```python
from build123d import *

# Parameters (mm, degrees)
F1_DEPTH  = 70
F3_DEPTH  = 10
F4_R      = 6.5
F4_R_2    = 3.35
F5_DEPTH  = 4.1439934524
F6_R      = 6.5
F6_R_2    = 3.35
F7_DEPTH  = 4.1439934524
F8_R      = 6.5
F8_R_2    = 3.35
F9_DEPTH  = 4.1439934524
F10_R     = 6.5
F10_R_2   = 3.35
F11_DEPTH = 4.1439934524
F12_R     = 5
F12_R_2   = 4.1
F13_DEPTH = 10


with BuildPart() as f1:
    # F0 (on Top) → F1 (new body)
    with BuildSketch(Plane.XY):
        with BuildLine():
            Line((17.5, 66.7439135802), (-17.5, 66.7439135802))
            ThreePointArc((-17.5, 66.7439135802), (-48.7903679019, 48.7903679019), (-66.7439135802, 17.5))
            Line((-66.7439135802, 17.5), (-66.7439135802, -17.5))
            ThreePointArc((-66.7439135802, -17.5), (-48.7903679019, -48.7903679019), (-17.5, -66.7439135802))
            Line((-17.5, -66.7439135802), (17.5, -66.7439135802))
            ThreePointArc((17.5, -66.7439135802), (48.7903679019, -48.7903679019), (66.7439135802, -17.5))
            Line((66.7439135802, -17.5), (66.7439135802, 17.5))
            ThreePointArc((66.7439135802, 17.5), (48.7903679019, 48.7903679019), (17.5, 66.7439135802))
        make_face()
        with BuildLine():
            ThreePointArc((-62.5999201277, 17.5), (-45.9619407771, 45.9619407771), (-17.5, 62.5999201277))
            Line((-17.5, 62.5999201277), (17.5, 62.5999201277))
            ThreePointArc((17.5, 62.5999201277), (45.9619407771, 45.9619407771), (62.5999201277, 17.5))
            Line((62.5999201277, 17.5), (62.5999201277, -17.5))
            ThreePointArc((62.5999201277, -17.5), (45.9619407771, -45.9619407771), (17.5, -62.5999201277))
            Line((17.5, -62.5999201277), (-17.5, -62.5999201277))
            ThreePointArc((-17.5, -62.5999201277), (-45.9619407771, -45.9619407771), (-62.5999201277, -17.5))
            Line((-62.5999201277, -17.5), (-62.5999201277, 17.5))
        make_face(mode=Mode.SUBTRACT)
    extrude(amount=F1_DEPTH)

    # F2 (on face) → F3 (join)
    with BuildSketch(Plane.XY.offset(70)):
        with BuildLine():
            Line((17.5, 71.3862731903), (-17.5, 71.3862731903))
            ThreePointArc((-17.5, 71.3862731903), (-51.9723484172, 51.9723484172), (-71.3862731903, 17.5))
            Line((-71.3862731903, 17.5), (-71.3862731903, -17.5))
            ThreePointArc((-71.3862731903, -17.5), (-51.9723484172, -51.9723484172), (-17.5, -71.3862731903))
            Line((-17.5, -71.3862731903), (17.5, -71.3862731903))
            ThreePointArc((17.5, -71.3862731903), (51.9723484172, -51.9723484172), (71.3862731903, -17.5))
            Line((71.3862731903, -17.5), (71.3862731903, 17.5))
            ThreePointArc((71.3862731903, 17.5), (51.9723484172, 51.9723484172), (17.5, 71.3862731903))
        make_face()
    extrude(amount=F3_DEPTH)

    # F4 (on face) → F5 (cut, through all)
    with BuildSketch(Plane.XZ.offset(66.7439135802)):
        with Locations((0, 53)):
            Circle(F4_R)
        with Locations((0, 34)):
            Circle(F4_R_2)
        with Locations((0, 17)):
            Circle(F4_R_2)
    extrude(amount=-F5_DEPTH, mode=Mode.SUBTRACT)

    # F6 (on face) → F7 (cut, through all)
    with BuildSketch(Plane.YZ.offset(66.7439135802)):
        with Locations((0, 53)):
            Circle(F6_R)
        with Locations((0, 34)):
            Circle(F6_R_2)
        with Locations((0, 17)):
            Circle(F6_R_2)
    extrude(amount=-F7_DEPTH, mode=Mode.SUBTRACT)

    # F8 (on face) → F9 (cut, through all)
    with BuildSketch(Plane(origin=(0, 66.7439135802, 0), x_dir=(-1, 0, 0), z_dir=(0, 1, 0))):
        with Locations((0, 53)):
            Circle(F8_R)
        with Locations((0, 34)):
            Circle(F8_R_2)
        with Locations((0, 17)):
            Circle(F8_R_2)
    extrude(amount=-F9_DEPTH, mode=Mode.SUBTRACT)

    # F10 (on face) → F11 (cut, through all)
    with BuildSketch(Plane(origin=(-66.7439135802, 0, 0), x_dir=(0, -1, 0), z_dir=(-1, 0, 0))):
        with Locations((0, 53)):
            Circle(F10_R)
        with Locations((0, 34)):
            Circle(F10_R_2)
        with Locations((0, 17)):
            Circle(F10_R_2)
    extrude(amount=-F11_DEPTH, mode=Mode.SUBTRACT)

    # F12 (on face) → F13 (cut, through all)
    with BuildSketch(Plane.XY.offset(80)):
        Circle(F12_R)
        with Locations((-42, 42)):
            Circle(F12_R_2)
        with Locations((42, 42)):
            Circle(F12_R_2)
        with Locations((42, -42)):
            Circle(F12_R_2)
        with Locations((-42, -42)):
            Circle(F12_R_2)
    extrude(amount=-F13_DEPTH, mode=Mode.SUBTRACT)


solid = f1.part
```
The model under review builds one solid part; all positions refer to its coordinate system, in mm. A direction names the side the tool comes from. Round coordinates to 2 decimals unless told otherwise and drop trailing zeros. Order: outer loops, then holes, each group sorted by start corner. A loop starts at its lowest first (then second) coordinate and runs counter-clockwise, first axis right, second up. Notation, with made-up numbers: (72.25, 53) -> (115.25, 53) arc R17 cw to (115.25, 75) -> close; hole circle Ø11 at (-24.5, 46). An arc over 180 degrees is marked (long way). One line per item, written item: value. Start each with the question number.
Q1. Take a section at A-A (z = 8). Write out the cut boundary in (x, y).
Q2. Machinability: for faces 5 (the face through (-4, 66.744, 35)), 6 (the face through (-49.15, -48.43, 34.51)), 7 (the face through (-1, 15, 70)), which of the approach directions +Z, -Z, +X, -X, +Y, -Y give a long, thin tool a straight path to every point of the face, cutting with its end or side? Answer none if there is none.
Q3. Wall thickness on line 1 (Z direction, x = 0, y = 65.7); line 2 (X direction, y = -1.5, z = 29): over which ranges is each line inside the solid? List them lowest first.
Q4. Mouldability with a two-part tool opening along X and no side actions: class faces 1 (the face through (64.7, -0.73, 30.73)), 2 (the face through (-51.57, 52.37, 74.93)), 3 (the face through (66.744, 4, 35)), 4 (the face through (-1.409, -64.701, 46.655)) as released by +X, released by -X, zero draft, split by the parting line, or undercut.
Q5. Take a section at D-D (y = 42). Write out the cut boundary in (x, z), and give its area (3 significant figures).
Q6. Take a section at C-C (z = 53). Count the separate pieces of the cut face and the enclosed holes in it, and give its area (3 significant figures).
Q7. Clearance check with flat-ended pins moving along their axes: pin 1 Ø10 at (y, z) = (16.5, 59) entering from -X; pin 2 Ø3 at (x, z) = (46, 50.5) entering from -Y; pin 3 Ø1.5 at (y, z) = (-39, 55) entering from +X; pin 4 Ø13 at (x, y) = (-42, 42) entering from -Z. State where each tip first meets the part, or that it passes through.
Q8. Take a section at B-B (y = 9). Write out the cut boundary in (x, z).
Reported:
1. outline: (-66.74, -17.5) arc R69 ccw to (-17.5, -66.74) -> (17.5, -66.74) arc R69 ccw to (66.74, -17.5) -> (66.74, 17.5) arc R69 ccw to (17.5, 66.74) -> (-17.5, 66.74) arc R69 ccw to (-66.74, 17.5) -> close; hole (-62.6, -17.5) arc R65 ccw to (-17.5, -62.6) -> (17.5, -62.6) arc R65 ccw to (62.6, -17.5) -> (62.6, 17.5) arc R65 ccw to (17.5, 62.6) -> (-17.5, 62.6) arc R65 ccw to (-62.6, 17.5) -> close
2. face 5: -Z, +X, -X, +Y
2. face 6: -Z, -X, -Y
2. face 7: -Z
3. line 1: z = 0 to 13.65, 20.35 to 30.65, 37.35 to 46.5, 59.5 to 80
3. line 2: x = -66.74 to -62.6, 62.6 to 66.74
4. face 1: zero draft
4. face 2: released by -X
4. face 3: released by +X
4. face 4: undercut
5. outline: (-60.32, 70) -> (-54.74, 70) -> (-54.74, 0) -> (-49.61, 0) -> (-49.61, 70) -> (-46.1, 70) -> (-46.1, 80) -> (-60.32, 80) -> close; (-37.9, 70) -> (37.9, 70) -> (37.9, 80) -> (-37.9, 80) -> close; (46.1, 70) -> (49.61, 70) -> (49.61, 0) -> (54.74, 0) -> (54.74, 70) -> (60.32, 70) -> (60.32, 80) -> (46.1, 80) -> close
5. area: 1,760 mm2
6. separate pieces: 4
6. enclosed holes: 0
6. area: 1,480 mm2
7. pin 1: stops at x = -66.74
7. pin 2: stops at y = -52.73
7. pin 3: stops at x = 57.43
7. pin 4: stops at z = 0
8. outline: (-71.39, 70) -> (-66.74, 70) -> (-66.74, 0) -> (-62.6, 0) -> (-62.6, 70) -> (62.6, 70) -> (62.6, 0) -> (66.74, 0) -> (66.74, 70) -> (71.39, 70) -> (71.39, 80) -> (-71.39, 80) -> close
